Read the model definition and answer for the solid it produces. Units are mm, in the model's axes. Face numbers are marked on the shaded views. A direction names the side the tool comes from. Round coordinates to 2 decimals unless told otherwise and drop trailing zeros. Write each loop counter-clockwise with the first axis right and the second up, starting at its lowest first coordinate (ties: lowest second). Pieces come first, ordered by that corner, then holes. Notation, with made-up numbers: (60, 61) - (66, 61) arc R26 cw to (66, 84) - close; hole circle Ø7 at (27.25, -16). An arc over 180 degrees is marked (long way). One line per item, written item: value. Start each with the question number.
(1) A cutting plane is placed at C-C, the plane y = 12.5. Determine the outline of the cut face in (x, z) (3 decimals), plus the area to 3 significant figures.
(2) The mould has two halves that part along Z. Classify the marked faces 4, 5, 6 and 7: +Z half, -Z half, draft (parallel to the pull), parting line (faces both ways), or undercut.
(3) A cutting plane is placed at A-A, the plane z = -36. Determine the outline of the cut face in (x, y) (3 decimals), plus the area to 3 significant figures.
(4) A cutting plane is placed at D-D, the plane x = 91.5. Determine the outline of the cut face in (y, z).
(5) For the marked faces 1, 2 and 3, determine the directions among +Z, -Z, +X, -X, +Y, -Y from which every point of the face is accessible in a straight line to the end or side of a thin tool.
(6) Find the intervals of material crossed by L1, parallel to X at y = 10, z = -34.5 (3 decimals); L2, parallel to Z at x = 48.5, y = 3; L3, parallel to X at y = 13.5, z = -29.5 (3 decimals), in increasing order.
(7) Flat-ended cylindrical pins translate along their axes: pin 1 Ø12 at (y, z) = (21.5, -20) entering from -X; pin 2 Ø3.5 at (y, z) = (9, -38) entering from +X; pin 3 Ø3 at (x, z) = (32.5, -32.5) entering from -Y; pin 4 Ø16.5 at (x, y) = (34.5, 15.5) entering from -Z. Find the tip coordinate at first contact, or state that the pin passes through.
(8) A cutting plane is placed at B-B, the plane x = 58.5. Determine the outline of the cut face in (y, z).
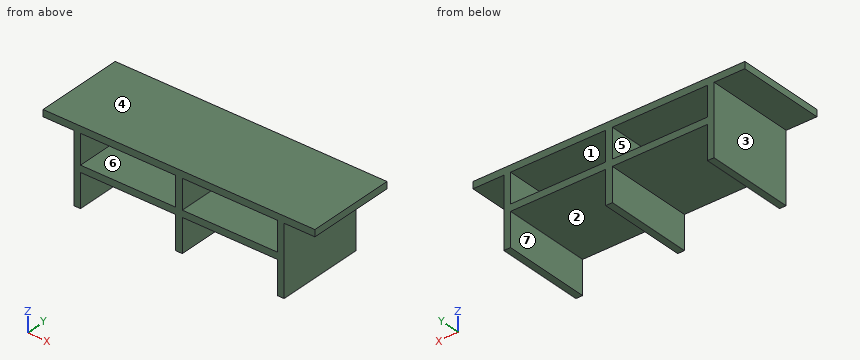
from build123d import *

# Parameters (mm, degrees)
SKETCH1_W           = 101
SKETCH1_H           = 43
BOSS_EXTRUDE1_DEPTH = 32.9
SKETCH4_W           = 101
SKETCH4_H           = 14.656
SKETCH4_W_2         = 11.451
SKETCH4_H_2         = 25.844
SKETCH4_W_3         = 11.445
SKETCH4_W_4         = 35.302
SKETCH4_H_3         = 12.422
SKETCH4_H_4         = 10.922
CUT_EXTRUDE2_DEPTH  = 32.9


with BuildPart() as part:
    # Sketch1 → Boss-Extrude1 (new body)
    with BuildSketch(Plane(origin=(0, 0, 0), x_dir=(1, 0, 0), z_dir=(0, 1, 0))):
        with Locations((50.5, 21.5)):
            Rectangle(SKETCH1_W, SKETCH1_H)
    extrude(amount=BOSS_EXTRUDE1_DEPTH)

    # Sketch4 → Cut-Extrude2 (cut)
    with BuildSketch(Plane(origin=(0, 32.9, 0), x_dir=(1, 0, 0), z_dir=(0, 1, 0))):
        with Locations((50.5, 7.328)):
            Rectangle(SKETCH4_W, SKETCH4_H)
        with Locations((95.2745, 30.078)):
            Rectangle(SKETCH4_W_2, SKETCH4_H_2)
        with Locations((5.7225, 30.078)):
            Rectangle(SKETCH4_W_3, SKETCH4_H_2)
        with Locations((31.596, 36.789)):
            Rectangle(SKETCH4_W_4, SKETCH4_H_3)
        with Locations((69.398, 36.789)):
            Rectangle(SKETCH4_W_4, SKETCH4_H_3)
        with Locations((69.398, 22.617)):
            Rectangle(SKETCH4_W_4, SKETCH4_H_4)
        with Locations((31.596, 22.617)):
            Rectangle(SKETCH4_W_4, SKETCH4_H_4)
    extrude(amount=-CUT_EXTRUDE2_DEPTH, mode=Mode.SUBTRACT)


solid = part.part
Here are the results:
1. outline: (0, -17.156) - (11.445, -17.156) - (11.445, -43) - (13.945, -43) - (13.945, -30.578) - (49.247, -30.578) - (49.247, -43) - (51.747, -43) - (51.747, -30.578) - (87.049, -30.578) - (87.049, -43) - (89.549, -43) - (89.549, -17.156) - (101, -17.156) - (101, -14.656) - (0, -14.656) - close; hole (13.945, -28.078) - (49.247, -28.078) - (49.247, -17.156) - (13.945, -17.156) - close; hole (51.747, -28.078) - (87.049, -28.078) - (87.049, -17.156) - (51.747, -17.156) - close
1. area: 623 mm²
2. face 4: +Z half
2. face 5: undercut
2. face 6: undercut
2. face 7: draft
3. outline: (11.445, 0) - (13.945, 0) - (13.945, 32.9) - (11.445, 32.9) - close; (49.247, 0) - (51.747, 0) - (51.747, 32.9) - (49.247, 32.9) - close; (87.049, 0) - (89.549, 0) - (89.549, 32.9) - (87.049, 32.9) - close
3. area: 247 mm²
4. outline: (0, -17.16) - (32.9, -17.16) - (32.9, -14.66) - (0, -14.66) - close
5. face 1: +Y, -Y
5. face 2: -Z, +Y, -Y
5. face 3: -Z, -X, +Y, -Y
6. L1: 11.445 to 13.945, 49.247 to 51.747, 87.049 to 89.549
6. L2: -30.58 to -28.08, -17.16 to -14.66
6. L3: 11.445 to 89.549
7. pin 1: x = 0
7. pin 2: x = 89.55
7. pin 3: through
7. pin 4: z = -30.58
8. outline: (0, -30.58) - (32.9, -30.58) - (32.9, -28.08) - (0, -28.08) - close; (0, -17.16) - (32.9, -17.16) - (32.9, -14.66) - (0, -14.66) - close
